The drawing under review shows one solid part. Ordinate dimensions are in mm from its lowest x, y, z. Give positions to 0.01 mm unless a question says otherwise; leave off trailing zeros. Write each loop counter-clockwise with the first axis right and the second up, starting at its lowest first coordinate (ties: lowest second). Pieces come first, ordered by that corner, then holes.
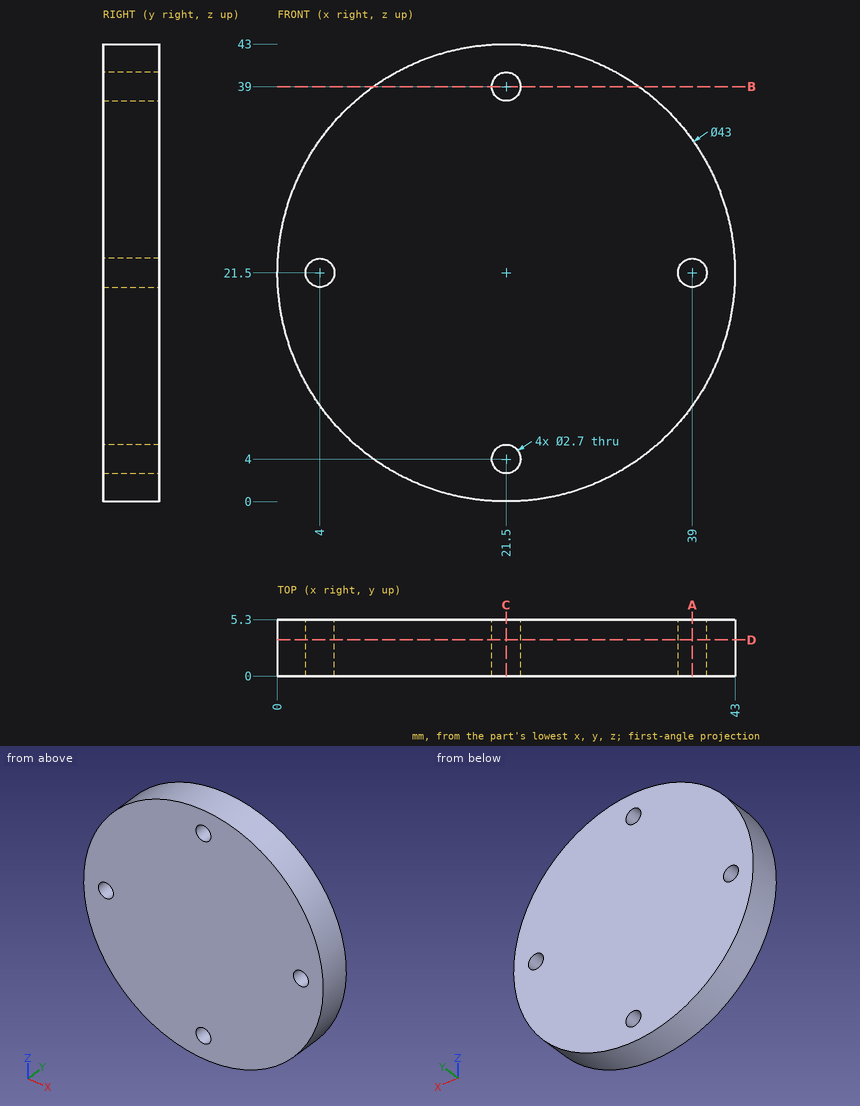
1) Insertion check: pin 1 (1 mm diameter, centred on x = 26, y = 3, fed in from +Z); pin 2 (1 mm diameter, centred on x = 10, y = 2.5, fed in from +Z). Each pin has a flat end and moves straight along its axis. Give the tip position at first contact, or say it passes through.
2) Consider section B-B, the plane z = 39. Give the boundary of the cut face in (x, y).
3) To check wall thickness, follow probe 1 along X at (y, z) = (1.4, 21.5); probe 2 along Z at (x, y) = (3.5, 4.65); probe 3 along X at (y, z) = (1.7, 4). State the ranges of each line that lie inside material, in increasing order.
4) Consider section A-A, the plane x = 39. Give the boundary of the cut face in (y, z), then the cut area to 3 significant figures.
5) Consider section D-D, the plane y = 3.4. Give the boundary of the cut face in (x, z).
6) Consider section C-C, the plane x = 21.5. Give the boundary of the cut face in (y, z), then the cut area to 3 significant figures.
Answer block:
1. pin 1: stops at z = 42.62
1. pin 2: stops at z = 39.97
2. outline: (9.01, 0) - (20.15, 0) - (20.15, 5.3) - (9.01, 5.3) - close; (22.85, 0) - (33.99, 0) - (33.99, 5.3) - (22.85, 5.3) - close
3. probe 1: x = 0 to 2.65, 5.35 to 37.65, 40.35 to 43
3. probe 2: z = 9.74 to 20.25, 22.75 to 33.26
3. probe 3: x = 9.01 to 20.15, 22.85 to 33.99
4. outline: (0, 9.01) - (5.3, 9.01) - (5.3, 20.15) - (0, 20.15) - close; (0, 22.85) - (5.3, 22.85) - (5.3, 33.99) - (0, 33.99) - close
4. area: 118 mm2
5. outline: circle Ø43 at (21.5, 21.5); hole circle Ø2.7 at (4, 21.5); hole circle Ø2.7 at (21.5, 4); hole circle Ø2.7 at (21.5, 39); hole circle Ø2.7 at (39, 21.5)
6. outline: (0, 0) - (5.3, 0) - (5.3, 2.65) - (0, 2.65) - close; (0, 5.35) - (5.3, 5.35) - (5.3, 37.65) - (0, 37.65) - close; (0, 40.35) - (5.3, 40.35) - (5.3, 43) - (0, 43) - close
6. area: 199 mm2
